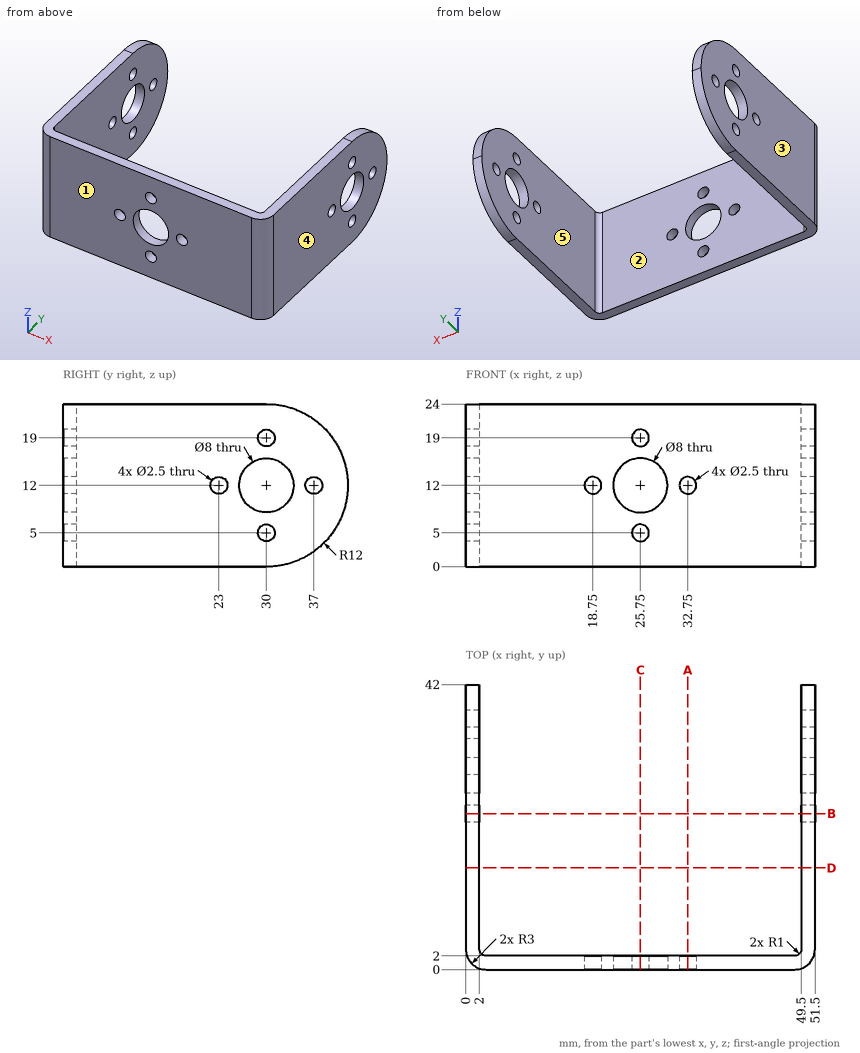
Check sheet for the drawn part. Datum: minimum x, y, z corner. Units: mm. A direction names the side the tool comes from. Coordinates: 2 decimals unless noted, no trailing zeros. Loops run counter-clockwise (first coordinate to the right, second up) from the corner with the lowest first, then second, coordinate; pieces in that order, holes last. Notation, with made-up numbers: (-37, 17.5) -> (-31, 17.5) arc R25 cw to (-31, 32.5) -> close; hole circle Ø1 at (57, 61.5). An arc over 180 degrees is marked (long way). Write each question's results on one line, items separated by ' | '.
Item 1: Material ranges on L1, parallel to X at y = 20.5, z = 6.25; L2, parallel to Y at x = 50.2, z = 12; L3, parallel to Y at x = 34, z = 21, recorded low to high.
Found:
L1: x = 0 to 2, 49.5 to 51.5 | L2: y = 0.53 to 21.75, 24.25 to 26, 34 to 35.75, 38.25 to 42 | L3: y = 0 to 2
Item 2: Section check D-D, the plane y = 15. Enter the section's corners in (x, z).
Found:
outline: (0, 0) -> (2, 0) -> (2, 24) -> (0, 24) -> close; (49.5, 0) -> (51.5, 0) -> (51.5, 24) -> (49.5, 24) -> close
Item 3: Section check A-A, the plane x = 32.75. Enter the section's corners in (y, z), plus the area to 3 significant figures.
Found:
outline: (0, 0) -> (2, 0) -> (2, 10.75) -> (0, 10.75) -> close; (0, 13.25) -> (2, 13.25) -> (2, 24) -> (0, 24) -> close | area: 43.0 mm2
Item 4: Section check C-C, the plane x = 25.75. Enter the section's corners in (y, z), plus the area to 3 significant figures.
Found:
outline: (0, 0) -> (2, 0) -> (2, 3.75) -> (0, 3.75) -> close; (0, 6.25) -> (2, 6.25) -> (2, 8) -> (0, 8) -> close; (0, 16) -> (2, 16) -> (2, 17.75) -> (0, 17.75) -> close; (0, 20.25) -> (2, 20.25) -> (2, 24) -> (0, 24) -> close | area: 22.0 mm2
Item 5: Gauge pin test, flat end, axial feed: pin 1 (13 mm diameter, centred on x = 25.75, z = 12, fed in from +Y). Record the tip position at first contact, or that the pin passes through.
Found:
pin 1: stops at y = 2
Item 6: Mould release check, pull along X, two halves, no side actions. Record for the marked faces 1, 2 and 3: +X half, -X half, draft (parallel to the pull), parting line (faces both ways), or undercut.
Found:
face 1: draft | face 2: undercut | face 3: -X half
Item 7: Section check B-B, the plane y = 23. Enter the section's corners in (x, z), plus the area to 3 significant figures.
Found:
outline: (0, 0) -> (2, 0) -> (2, 10.75) -> (0, 10.75) -> close; (0, 13.25) -> (2, 13.25) -> (2, 24) -> (0, 24) -> close; (49.5, 0) -> (51.5, 0) -> (51.5, 10.75) -> (49.5, 10.75) -> close; (49.5, 13.25) -> (51.5, 13.25) -> (51.5, 24) -> (49.5, 24) -> close | area: 86.0 mm2
Item 8: Tool access check on the marked faces 4 and 5. Record the directions out of +Z, -Z, +X, -X, +Y, -Y that give a thin tool (end or side, any length) a straight path to the whole face; none if there is none.
Found:
face 4: +Z, -Z, +X, +Y, -Y | face 5: +Z, -Z, +Y
